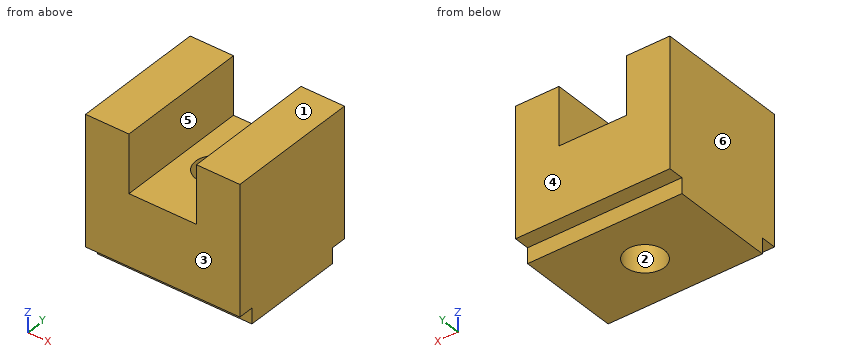
```python
from build123d import *

# Parameters (mm, degrees)
SKETCH1_W               = 25.4
SKETCH1_H               = 22.098
SKETCH1_R               = 3.175
BOSS_EXTRUDE1_DEPTH     = 23.749
SKETCH2_W               = 11.1125
SKETCH2_H               = 22.098
CUT_EXTRUDE1_DEPTH      = 9.525
CUT_EXTRUDE2_DEPTH      = 30.109884953
CUT_EXTRUDE2_DEPTH_BACK = 30.109884953
SKETCH3_W               = 2.54
SKETCH3_H               = 2.54


with BuildPart() as part:
    # Sketch1 → Boss-Extrude1 (new body)
    with BuildSketch(Plane.XY):
        Rectangle(SKETCH1_W, SKETCH1_H)
        with Locations(Location((0, 0, 0), (0, 0, 180))):
            Circle(SKETCH1_R, mode=Mode.SUBTRACT)
    extrude(amount=BOSS_EXTRUDE1_DEPTH)

    # Sketch2 → Cut-Extrude1 (cut)
    with BuildSketch(Plane.XY.offset(23.749)):
        Rectangle(SKETCH2_W, SKETCH2_H)
    extrude(amount=-CUT_EXTRUDE1_DEPTH, mode=Mode.SUBTRACT)

    # Sketch3 → Cut-Extrude2 (cut, two sides: drawn at the far end of the back side and taken through both)
    with BuildSketch(Plane(origin=(0, 0, 0), x_dir=(0, 0, -1), z_dir=(1, 0, 0)).offset(-CUT_EXTRUDE2_DEPTH_BACK)):
        with Locations((-1.27, 9.779)):
            Rectangle(SKETCH3_W, SKETCH3_H)
        with Locations((-1.27, -9.779)):
            Rectangle(SKETCH3_W, SKETCH3_H)
    extrude(amount=CUT_EXTRUDE2_DEPTH + CUT_EXTRUDE2_DEPTH_BACK, mode=Mode.SUBTRACT)


solid = part.part
```
Source: CAD feature listing. Evaluate the final solid. Frame: model axes, mm. Face numbers are marked on the shaded views. A direction names the side the tool comes from. Give positions to 0.01 mm unless a question says otherwise; leave off trailing zeros. Loops run counter-clockwise (first coordinate to the right, second up) from the corner with the lowest first, then second, coordinate; pieces in that order, holes last. Notation, with made-up numbers: (65.5, 51.5) -> (94.5, 51.5) arc R4 cw to (94.5, 55.5) -> close; hole circle Ø11 at (5, -12). An arc over 180 degrees is marked (long way). Use a Markdown table: item, result. Add a question column.
(1) Section query B-B (x = 0). Output: boundary loops of the cut face in (y, z) (3 decimals), then the cut area to 3 significant figures.
(2) Section query C-C (z = 11.75). Output: boundary loops of the cut face in (x, y) (3 decimals), then the cut area to 3 significant figures.
(3) First-contact query: pin 1 Ø6 at (x, z) = (-2, 19.5) entering from +Y; pin 2 Ø1.3 at (x, y) = (-4.5, 9.5) entering from -Z; pin 3 Ø2 at (x, z) = (4, 1) entering from -Y; pin 4 Ø0.8 at (x, z) = (2.5, 2) entering from +Y. Flat tips, straight axial feed; report the tip coordinate or a pass-through.
(4) Pull-direction query (Y, two-part tool) for the marked faces 1, 2, 3 and 4; classes: +Y half, -Y half, draft (parallel to the pull), parting line (faces both ways), or undercut.
(5) Ray query, line 1 (Y direction, x = 0, z = 5.25) (3 decimals); line 2 (X direction, y = -2.75, z = 15.5); line 3 (Z direction, x = 4.5, y = -6.75). Return the intervals inside material, ascending.
(6) Access query for the marked faces 5 and 6. Directions: +Z, -Z, +X, -X, +Y, -Y. A direction counts if a zero-diameter tool reaches every point of the face in a straight line with its end or side. Return the directions, or none.
(7) Section query A-A (y = 0). Output: boundary loops of the cut face in (x, z) (3 decimals), then the cut area to 3 significant figures.
(8) Section query D-D (z = 21.75). Output: boundary loops of the cut face in (x, y), then the cut area to 3 significant figures.
Checked values:
| question | item | result |
|---|---|---|
| 1 | outline | (-11.049, 2.54) -> (-8.509, 2.54) -> (-8.509, 0) -> (-3.175, 0) -> (-3.175, 14.224) -> (-11.049, 14.224) -> close; (3.175, 0) -> (8.509, 0) -> (8.509, 2.54) -> (11.049, 2.54) -> (11.049, 14.224) -> (3.175, 14.224) -> close |
| 1 | area | 211 mm^2 |
| 2 | outline | (-12.7, -11.049) -> (12.7, -11.049) -> (12.7, 11.049) -> (-12.7, 11.049) -> close; hole circle Ø6.35 at (0, 0) |
| 2 | area | 530 mm^2 |
| 3 | pin 1 | through |
| 3 | pin 2 | z = 2.54 |
| 3 | pin 3 | y = -8.51 |
| 3 | pin 4 | y = 8.51 |
| 4 | face 1 | draft |
| 4 | face 2 | undercut |
| 4 | face 3 | -Y half |
| 4 | face 4 | +Y half |
| 5 | line 1 | -11.049 to -3.175, 3.175 to 11.049 |
| 5 | line 2 | -12.7 to -5.56, 5.56 to 12.7 |
| 5 | line 3 | 0 to 14.22 |
| 6 | face 5 | +Z, +Y, -Y |
| 6 | face 6 | +Z, -Z, -X, +Y, -Y |
| 7 | outline | (-12.7, 0) -> (-3.175, 0) -> (-3.175, 14.224) -> (-5.556, 14.224) -> (-5.556, 23.749) -> (-12.7, 23.749) -> close; (3.175, 0) -> (12.7, 0) -> (12.7, 23.749) -> (5.556, 23.749) -> (5.556, 14.224) -> (3.175, 14.224) -> close |
| 7 | area | 407 mm^2 |
| 8 | outline | (-12.7, -11.05) -> (-5.56, -11.05) -> (-5.56, 11.05) -> (-12.7, 11.05) -> close; (5.56, -11.05) -> (12.7, -11.05) -> (12.7, 11.05) -> (5.56, 11.05) -> close |
| 8 | area | 316 mm^2 |
